Work out the finished part from the listing and answer in its coordinate system (mm). Face numbers are marked on the shaded views. A direction names the side the tool comes from. Coordinates: 2 decimals unless noted, no trailing zeros. Write each loop counter-clockwise with the first axis right and the second up, starting at its lowest first coordinate (ties: lowest second). Pieces come first, ordered by that corner, then holes. Notation, with made-up numbers: (-13.75, 44) - (9.25, 44) arc R16 cw to (9.25, 53) - close; hole circle Ø8 at (-38, 26). An arc over 180 degrees is marked (long way). One line per item, written item: value.
Autodesk Inventor part; units mm, degrees
ref_plane "ROD_BA_XY" through (10, 0, 0) normal (-1, 0, 0) x (0, 0, -1)
ref_plane "ROD_BA_YZ" through (10, 0, 0) normal (0, 0, -1) x (0, -1, 0)
ref_plane "ROD_BA_ZX" through (10, 0, 0) normal (0, -1, 0) x (-1, 0, 0)
sketch "Sketch_5" plane through (0, 0, 0) normal (0, 0, 1) x (1, 0, 0)
  line L0 (105.5, 0) -> (0, 0)
  line L1 (0, 0) -> (0, 2.0095)
  line L2 (0, 2.0095) -> (0.4905, 2.5)
  line L3 (0.4905, 2.5) -> (15, 2.5)
  line L4 (15, 2.5) -> (15, 2.067)
  line L5 (15, 2.067) -> (16.5, 2.067)
  line L6 (16.5, 2.067) -> (16.5, 2.5)
  line L7 (16.5, 2.5) -> (100.5, 2.5)
  line L8 (100.5, 2.5) -> (100.5, 8)
  line L9 (100.5, 8) -> (105.5, 8)
  line L10 (105.5, 8) -> (105.5, 0)
  line L11 (105.5, 0) -> (0, 0)
revolve "Revolution1" add sketch "Sketch_5" angle 360 about axis through (105.5, 0, 0) along (1, 0, 0)
thread "Thread1"
ref_plane "ROD_BA_XY" through (10, 0, 0) normal (-1, 0, 0) x (0, 0, -1)
ref_plane "ROD_BA_YZ" through (10, 0, 0) normal (0, 0, -1) x (0, -1, 0)
ref_plane "ROD_BA_ZX" through (10, 0, 0) normal (0, -1, 0) x (-1, 0, 0)
ref_plane "ROD_BODY_XY" through (28, 0, 0) normal (-1, 0, 0) x (0, 0, -1)
ref_plane "ROD_BODY_YZ" through (28, 0, 0) normal (0, 0, -1) x (0, -1, 0)
ref_plane "ROD_BODY_ZX" through (28, 0, 0) normal (0, -1, 0) x (-1, 0, 0)
ref_plane "rodnt1_XY" through (7.5, 0, 0) normal (1, 0, 0) x (0, 0, -1)
ref_plane "rodnt1_YZ" through (7.5, 0, 0) normal (0, 0, -1) x (0, 1, 0)
ref_plane "rodnt1_ZX" through (7.5, 0, 0) normal (0, 1, 0) x (1, 0, 0)
properties part number "CJ2B16-60Z_ROD" material "ステンレス鋼"
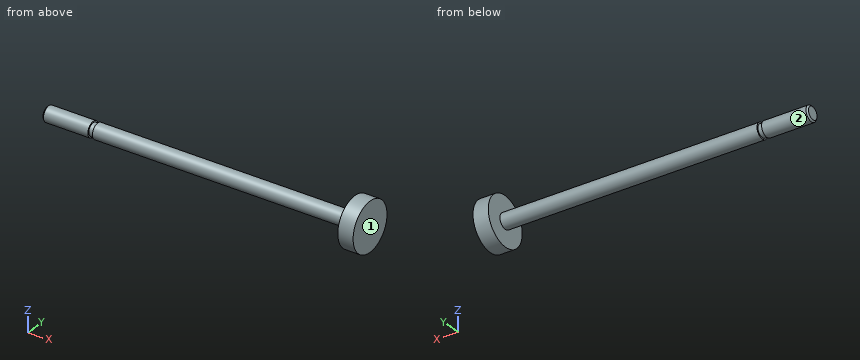
Item 1: Which of the six approach directions +Z, -Z, +X, -X, +Y, -Y give full straight-line access (tool end or side, diameter ignored) to the marked faces 1 and 2?
Evaluation:
face 1: +Z, -Z, +X, +Y, -Y
face 2: -X
Item 2: Section C-C, the plane x = 50.5 is taken. Determine the outline of the cut face in (y, z), then the cut area to 3 significant figures.
Evaluation:
outline: circle Ø5 at (0, 0)
area: 19.6 mm2
Item 3: Consider probe 1 along X at (y, z) = (5.25, 3); probe 2 along Y at (x, z) = (50, 1.5); probe 3 along X at (y, z) = (2, -0.75). Determine where each line is inside the solid, lowest interval first.
Evaluation:
probe 1: x = 100.5 to 105.5
probe 2: y = -2 to 2
probe 3: x = 0.13 to 15, 16.5 to 105.5
Item 4: Section A-A, the plane z = 0 is taken. Determine the outline of the cut face in (x, y), then the cut area to 3 significant figures.
Evaluation:
outline: (0, -2.01) - (0.49, -2.5) - (15, -2.5) - (15, -2.07) - (16.5, -2.07) - (16.5, -2.5) - (100.5, -2.5) - (100.5, -8) - (105.5, -8) - (105.5, 8) - (100.5, 8) - (100.5, 2.5) - (16.5, 2.5) - (16.5, 2.07) - (15, 2.07) - (15, 2.5) - (0.49, 2.5) - (0, 2.01) - close
area: 581 mm2
Item 5: Section D-D, the plane z = 4 is taken. Determine the outline of the cut face in (x, y).
Evaluation:
outline: (100.5, -6.93) - (105.5, -6.93) - (105.5, 6.93) - (100.5, 6.93) - close
Item 6: Given pin 1 (4 mm diameter, centred on x = 80.5, y = -2, fed in from +Z); pin 2 (1.5 mm diameter, centred on x = 26.5, y = 2.5, fed in from -Z); pin 3 (3 mm diameter, centred on x = 73, y = -3.5, fed in from +Z), each flat-ended and moving along its own axis, determine where each tip first touches the part or whether it passes through.
Evaluation:
pin 1: stops at z = 2.5
pin 2: stops at z = -1.79
pin 3: stops at z = 1.5
